Input: part model. Units: mm. Frame: model coordinates. Face numbers are marked on the shaded views. Give positions to 0.01 mm unless a question says otherwise; leave off trailing zeros. Loops run counter-clockwise (first coordinate to the right, second up) from the corner with the lowest first, then second, coordinate; pieces in that order, holes last. Notation, with made-up numbers: (53.5, 40.25) - (81.5, 40.25) arc R9 cw to (81.5, 47.25) - close; hole circle Ø5 at (80, -16.75). An arc over 180 degrees is marked (long way). Answer as a JSON object with one key per item and string values.
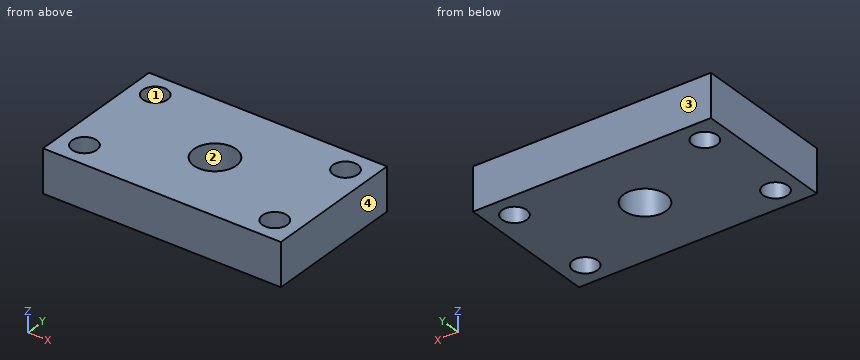
from build123d import *

# Parameters (mm, degrees)
F0_W     = 12.7
F0_H     = 7.62
F0_W_2   = 10.16
F0_H_2   = 5.08
F1_DEPTH = 2.286
F2_D     = 1.3208
F3_D     = 2.2606


with BuildPart() as f1:
    # F0 (on Top) → F1 (new body)
    with BuildSketch(Plane.XY):
        Rectangle(F0_W, F0_H)
        Rectangle(F0_W_2, F0_H_2, mode=Mode.SUBTRACT)
        Rectangle(F0_W_2, F0_H_2)
    extrude(amount=F1_DEPTH)

    # F2 (through all)
    with Locations(Plane(origin=(0, 0, 0), x_dir=(1, 0, 0), z_dir=(0, 0, -1))):
        with Locations((-5.08, -2.54), (5.08, -2.54), (5.08, 2.54), (-5.08, 2.54)):
            Hole(F2_D / 2)

    # F3 (through all)
    with Locations(Plane(origin=(0, 0, 0), x_dir=(1, 0, 0), z_dir=(0, 0, -1))):
        with Locations((0, 0)):
            Hole(F3_D / 2)


solid = f1.part
Item 1: Material intervals for line 1 (Y direction, x = -5.08, z = 0.75); line 2 (X direction, y = -2.54, z = 0.55); line 3 (X direction, y = 3, z = 1), sorted ascending. Write a range as [from, to].
Geometry check:
{"line 1": "y = [-3.81, -3.2], [-1.88, 1.88], [3.2, 3.81]", "line 2": "x = [-6.35, -5.74], [-4.42, 4.42], [5.74, 6.35]", "line 3": "x = [-6.35, -5.55], [-4.61, 4.61], [5.55, 6.35]"}
Item 2: Cut plane D-D (y = 1). Return loops of the section in (x, z).
Geometry check:
{"outline": "(-6.35, 0) - (-0.53, 0) - (-0.53, 2.29) - (-6.35, 2.29) - close; (0.53, 0) - (6.35, 0) - (6.35, 2.29) - (0.53, 2.29) - close"}
Item 3: Contact query for a flat-ended pin moving along its axis: P1, Ø2, axis at x = 4, y = -2, coming from the -Z side. Output: stop coordinate, or through.
Geometry check:
{"P1": "stops at z = 0"}
Item 4: Cut plane A-A (x = 5.08). Return loops of the section in (y, z).
Geometry check:
{"outline": "(-3.81, 0) - (-3.2, 0) - (-3.2, 2.29) - (-3.81, 2.29) - close; (-1.88, 0) - (1.88, 0) - (1.88, 2.29) - (-1.88, 2.29) - close; (3.2, 0) - (3.81, 0) - (3.81, 2.29) - (3.2, 2.29) - close"}
Item 5: Mould query, pull axis X, two halves, no side actions, for the marked faces 1, 2, 3 and 4. Classes: released by +X, released by -X, zero draft, split by the parting line, or undercut.
Geometry check:
{"face 1": "undercut", "face 2": "undercut", "face 3": "zero draft", "face 4": "released by +X"}
Item 6: Cut plane C-C (z = 1.3). Return loops of the section in (x, y).
Geometry check:
{"outline": "(-6.35, -3.81) - (6.35, -3.81) - (6.35, 3.81) - (-6.35, 3.81) - close; hole circle Ø1.32 at (-5.08, -2.54); hole circle Ø1.32 at (-5.08, 2.54); hole circle Ø2.26 at (0, 0); hole circle Ø1.32 at (5.08, -2.54); hole circle Ø1.32 at (5.08, 2.54)"}
Item 7: Cut plane B-B (y = 2.54). Return loops of the section in (x, z), then the cut area to 3 significant figures.
Geometry check:
{"outline": "(-6.35, 0) - (-5.74, 0) - (-5.74, 2.29) - (-6.35, 2.29) - close; (-4.42, 0) - (4.42, 0) - (4.42, 2.29) - (-4.42, 2.29) - close; (5.74, 0) - (6.35, 0) - (6.35, 2.29) - (5.74, 2.29) - close", "area": "23.0 mm2"}
